Could you check a few things on this model? Use its own coordinates, in mm. Face numbers are marked on the shaded views. Give positions to 0.01 mm unless a question says otherwise; leave off trailing zeros. Write each loop counter-clockwise with the first axis right and the second up, starting at its lowest first coordinate (ties: lowest second). Pieces come first, ordered by that corner, then holes. Notation, with made-up numbers: (4.25, 51.5) - (24.25, 51.5) arc R29 ccw to (24.25, 82.5) - close; hole circle Ø1 at (68.25, 86.25). An arc over 180 degrees is marked (long way). Answer as a JSON object with one key per item and string values. Group by question number.
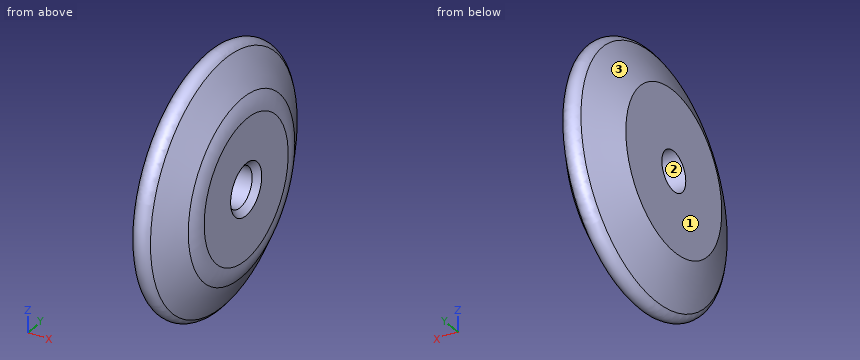
```python
from build123d import *

# Parameters (mm, degrees)
F0_W    = 30
F0_H    = 30
F7_R    = 5
F1_R    = 20
F2_SIZE = 3


# Not quite as in the source:
# - the program builds the solid bodies; features that only make, move or delete a surface that nothing else refers to are left out


with BuildPart() as f6:
    # F0 (on Front) → F6 (revolve)
    with BuildSketch(Plane.XZ):
        Polygon((-34.5531404018, 69.9733775854), (-48.6977283961, 39.9733775854), (-18.6977283961, 39.9733775854), align=None)
        with Locations((-33.6977283961, 24.9733775854)):
            Rectangle(F0_W, F0_H)
    revolve(axis=Axis((8.8008791208, 0, 0), (1, 0, 0)))

    # F7
    f7_edges = [f6.edges().sort_by_distance(p)[0] for p in [
        (-34.55314, 0, -69.973378),
    ]]
    fillet(f7_edges, radius=F7_R)

    # F1
    f1_edges = [f6.edges().sort_by_distance(p)[0] for p in [
        (-18.697728, 0, -39.973378),
    ]]
    fillet(f1_edges, radius=F1_R)

    # F2
    f2_edges = [f6.edges().sort_by_distance(p)[0] for p in [
        (-18.697728, 0, -9.973378),
    ]]
    chamfer(f2_edges, length=F2_SIZE)


solid = f6.part
```
(1) I need wall thicknesses on L1, parallel to Y at x = -34, z = 0; L2, parallel to Y at x = -27, z = 1.5; L3, parallel to Z at x = -42.5, y = -8. Which ranges of each line are inside material? Lowest first, please.
(2) I want a section at B-B, the plane x = -44. Please give me the cut outline in (y, z).
(3) I want a section at A-A, the plane x = -24. Please give me the cut outline in (y, z).
(4) If we mould it in two halves opening along Z, with no side actions, what happens to the marked faces 1, 2 and 3? For each: +Z half, -Z half, draft (parallel to the pull), parting line (faces both ways), or undercut.
(5) Will these pins go through, and if not, where does the flat tip stop? P1, Ø12, axis at x = -33.5, z = 33.5, coming from the -Y side; P2, Ø6, axis at y = -15.5, z = -44, coming from the -X side; P3, Ø12, axis at x = -36.5, z = -9.5, coming from the -Y side.
Entries:
{
 "1": {"L1": "-63.78 to -9.97, 9.97 to 63.78", "L2": "-55.66 to -9.86, 9.86 to 55.66", "L3": "-52.51 to -5.96, 5.96 to 52.51"},
 "2": {"outline": "circle Ø99.87 at (0, 0); hole circle Ø19.95 at (0, 0)"},
 "3": {"outline": "circle Ø100.01 at (0, 0); hole circle Ø19.95 at (0, 0)"},
 "4": {"face 1": "draft", "face 2": "undercut", "face 3": "parting line"},
 "5": {"P1": "y = -57.54", "P2": "x = -46.96", "P3": "y = -63.67"}
}
